Design review of the part built by this model. Coordinates are the model's own, in mm. A direction names the side the tool comes from. Coordinates: 2 decimals unless noted, no trailing zeros. Order: outer loops, then holes, each group sorted by start corner. A loop starts at its lowest first (then second) coordinate and runs counter-clockwise, first axis right, second up. Notation, with made-up numbers: (81, 65.25) -> (110, 65.25) arc R21 ccw to (110, 92.25) -> close; hole circle Ø1 at (43.25, 79.5). An arc over 180 degrees is marked (long way). Write item = value, one per line.
```python
from build123d import *

# Parameters (mm, degrees)
SKETCH1_R           = 12.62515314
BOSS_EXTRUDE1_DEPTH = 127.254
SKETCH2_W           = 21.600890372
SKETCH2_H           = 6.08719661
CUT_EXTRUDE1_DEPTH  = 155.702
CUT_EXTRUDE2_DEPTH  = 141.081655767
BOSS_EXTRUDE2_DEPTH = 12.755190121
BOSS_EXTRUDE3_DEPTH = 12.755190121
SKETCH6_R           = 2.435016118
CUT_EXTRUDE3_DEPTH  = 11.231190121
SKETCH7_R           = 2.472305811
CUT_EXTRUDE4_DEPTH  = 10.977190121


with BuildPart() as part:
    # Sketch1 → Boss-Extrude1 (new body)
    with BuildSketch(Plane(origin=(0, 0, 0), x_dir=(1, 0, 0), z_dir=(0, 1, 0))):
        with Locations(Location((0, 0, 0), (0, 0, 270))):
            Circle(SKETCH1_R)
    extrude(amount=-BOSS_EXTRUDE1_DEPTH)

    # Sketch2 → Cut-Extrude1 (cut)
    with BuildSketch(Plane(origin=(0, -127.254, 0), x_dir=(-1, 0, 0), z_dir=(0, -1, 0))):
        with Locations((0, -9.581554835)):
            Rectangle(SKETCH2_W, SKETCH2_H)
    extrude(amount=-CUT_EXTRUDE1_DEPTH, mode=Mode.SUBTRACT)

    # Sketch3 → Cut-Extrude2 (cut)
    with BuildSketch(Plane(origin=(0, -127.254, 0), x_dir=(-1, 0, 0), z_dir=(0, -1, 0))):
        with BuildLine():
            Line((3.126169088, 0), (-3.091625783, 0))
            ThreePointArc((-3.091625783, 0), (0.017271652, 3.108897435), (3.126169088, 0))
        make_face()
    extrude(amount=-CUT_EXTRUDE2_DEPTH, mode=Mode.SUBTRACT)

    # Sketch4 → Boss-Extrude2 (add)
    with BuildSketch(Plane.XZ.offset(127.254)):
        Polygon((-10.800445186, 6.53795653), (-8.274777075, 6.53795653), (-10.800445186, 20.396051451), (-13.364649969, 20.396051451), align=None)
    extrude(amount=-BOSS_EXTRUDE2_DEPTH)

    # Sketch5 → Boss-Extrude3 (add)
    with BuildSketch(Plane.XZ.offset(127.254)):
        Polygon((10.800445186, 6.53795653), (8.287884941, 6.53795653), (10.800445186, 20.258509361), (13.265579683, 20.258509361), align=None)
    extrude(amount=-BOSS_EXTRUDE3_DEPTH)

    # Sketch6 → Cut-Extrude3 (cut)
    with BuildSketch(Plane(origin=(9.324781226, 0, -1.67535814), x_dir=(-0.17683579611178707, 0, -0.9842403676000647), z_dir=(0.9842403676000648, 0, -0.17683579611178707))):
        with Locations((-15.314949053, -120.83230441)):
            Circle(SKETCH6_R)
    extrude(amount=-CUT_EXTRUDE3_DEPTH, mode=Mode.SUBTRACT)

    # Sketch7 → Cut-Extrude4 (cut)
    with BuildSketch(Plane(origin=(-9.273218408, 0, -1.715851358), x_dir=(-0.18194456837394912, 0, 0.9833087887531655), z_dir=(-0.9833087887531655, 0, -0.18194456837394912))):
        with Locations((16.069302572, -120.876404939)):
            Circle(SKETCH7_R)
    extrude(amount=-CUT_EXTRUDE4_DEPTH, mode=Mode.SUBTRACT)


solid = part.part
```
(1) Insertion check: pin 1 (3 mm diameter, centred on x = -3.5, y = -88, fed in from -Z); pin 2 (3 mm diameter, centred on x = 8.5, y = -88, fed in from -Z); pin 3 (12 mm diameter, centred on x = -7, y = -90.5, fed in from +Z). Each pin has a flat end and moves straight along its axis. Give the tip position at first contact, or say it passes through.
Report:
pin_1 = -12.47
pin_2 = -10.51
pin_3 = 6.54
(2) The part is to be moulded in two halves that separate along X. For faces 6 (the flat face through (-12.1, -123.8, 13.56)), 7 (the cylindrical face through (-11.19, -123.07, 15.43)), 8 (the flat face through (-12, -121, 20.396)), 9 (the cylindrical face through (0.37, -62.74, -12.62)), say which applies: released by +X, released by -X, zero draft, split by the parting line, or undercut.
Report:
face_6 = released by -X
face_7 = undercut
face_8 = zero draft
face_9 = split by the parting line
(3) For L1, parallel to X at y = -119.5, z = -2; L2, parallel to X at y = -99, z = -2.5; L3, parallel to Z at x = 1.25, y = -39, list the stretches that pass through material, from the lowest coordinate up.
Report:
L1 = -12.47 to -2.4, 2.36 to 12.47
L2 = -12.38 to -1.87, 1.83 to 12.38
L3 = -12.56 to -2.84, 0 to 6.54
(4) For faces 1 (the flat face through (0, -65, 0)), 2 (the flat face through (12, -121, 20.259)), 3 (the flat face through (12.05, -123.8, 13.49)), 4 (the flat face through (-11, -114.499, 14)), 5 (the flat face through (9.247, -122.383, 11.778)), list the 3-axis set-ups (+Z, -Z, +X, -X, +Y, -Y) from which the entire face can be reached by the end or side of a thin tool; tool diameter is ignored.
Report:
face_1 = +Y, -Y
face_2 = +Z, +X, +Y, -Y
face_3 = +X, +Y, -Y
face_4 = +Z, +X, -X, +Y
face_5 = +Z, +Y, -Y
(5) We need section A-A (x = 0). Write out the cut boundary in (y, z), and give its area (3 significant figures).
Report:
outline = (-127.25, -12.63) -> (0, -12.63) -> (0, -3.11) -> (-127.25, -3.11) -> close; (-127.25, 0) -> (0, 0) -> (0, 6.54) -> (-127.25, 6.54) -> close
area = 2,040 mm²
(6) We need section B-B (z = -2). Write out the cut boundary in (x, y), and give its area (3 significant figures).
Report:
outline = (-12.47, -127.25) -> (-2.4, -127.25) -> (-2.4, 0) -> (-12.47, 0) -> close; (2.36, -127.25) -> (12.47, -127.25) -> (12.47, 0) -> (2.36, 0) -> close
area = 2,570 mm²
(7) We need section C-C (y = -23). Write out the cut boundary in (x, z).
Report:
outline = (-10.8, 6.54) arc R12.63 ccw (long way) to (10.8, 6.54) -> close; hole (-3.13, 0) arc R3.11 ccw to (3.09, 0) -> close
(8) We need section D-D (z = 5). Write out the cut boundary in (x, y), and give its area (3 significant figures).
Report:
outline = (-11.59, -127.25) -> (11.59, -127.25) -> (11.59, 0) -> (-11.59, 0) -> close
area = 2,950 mm²
